Can you work these out from the model? Positions are in its coordinate system, mm. Face numbers are marked on the shaded views. Give positions to 0.01 mm unless a question says otherwise; leave off trailing zeros. Write each loop counter-clockwise with the first axis right and the second up, starting at its lowest first coordinate (ties: lowest second). Pieces come first, ordered by that corner, then holes.
from build123d import *

# Parameters (mm, degrees)
SKETCH1_R               = 17.5
BOSS_EXTRUDE1_DEPTH     = 15
SKETCH2_R               = 1.5
CUT_EXTRUDE1_DEPTH      = 3
CUT_EXTRUDE2_START      = -3
SKETCH3_R               = 1.5
CUT_EXTRUDE2_DEPTH      = 3
CUT_EXTRUDE3_DEPTH      = 0.2
CUT_EXTRUDE3_DEPTH_BACK = 0.2
SKETCH4_R               = 17.5
SKETCH4_R_2             = 16.5
CHAMFER1_SIZE           = 1
SKETCH5_R               = 2.5
CUT_EXTRUDE4_DEPTH      = 29.939592257


with BuildPart() as part:
    # Sketch1 → Boss-Extrude1 (new body)
    with BuildSketch(Plane(origin=(0, 0, 0), x_dir=(1, 0, 0), z_dir=(0, 1, 0))):
        with Locations(Location((0, 0, 0), (0, 0, 270))):
            Circle(SKETCH1_R)
    extrude(amount=BOSS_EXTRUDE1_DEPTH)

    # Sketch2 → Cut-Extrude1 (cut)
    with BuildSketch(Plane(origin=(0, 15, 0), x_dir=(1, 0, 0), z_dir=(0, 1, 0))):
        with Locations(Location((-8, 0, 0), (0, 0, 270))):
            Circle(SKETCH2_R)
        with Locations(Location((8, 0, 0), (0, 0, 270))):
            Circle(SKETCH2_R)
        with Locations(Location((0, 8, 0), (0, 0, 270))):
            Circle(SKETCH2_R)
        with Locations(Location((0, -8, 0), (0, 0, 270))):
            Circle(SKETCH2_R)
    extrude(amount=-CUT_EXTRUDE1_DEPTH, mode=Mode.SUBTRACT)

    # Sketch3 → Cut-Extrude2 (cut)
    with BuildSketch(Plane.XZ.offset(CUT_EXTRUDE2_START)):
        with Locations(Location((0, 9.5, 0), (0, 0, 270))):
            Circle(SKETCH3_R)
        with Locations(Location((0, -9.5, 0), (0, 0, 270))):
            Circle(SKETCH3_R)
        with Locations(Location((8, 0, 0), (0, 0, 90))):
            Circle(SKETCH3_R)
        with Locations(Location((-8, 0, 0), (0, 0, 90))):
            Circle(SKETCH3_R)
    extrude(amount=CUT_EXTRUDE2_DEPTH, mode=Mode.SUBTRACT)

    # Sketch4 → Cut-Extrude3 (cut, two sides: drawn at the far end of the back side and taken through both)
    with BuildSketch(Plane(origin=(0, 5, 0), x_dir=(-1, 0, 0), z_dir=(0, -1, 0)).offset(-CUT_EXTRUDE3_DEPTH_BACK)):
        with Locations(Location((0, 0, 0), (0, 0, 90))):
            Circle(SKETCH4_R)
        with Locations(Location((0, 0, 0), (0, 0, 90))):
            Circle(SKETCH4_R_2, mode=Mode.SUBTRACT)
    extrude(amount=CUT_EXTRUDE3_DEPTH + CUT_EXTRUDE3_DEPTH_BACK, mode=Mode.SUBTRACT)

    # Chamfer1
    chamfer1_edges = [part.edges().sort_by_distance(p)[0] for p in [
        (0, 0, -17.5),
        (0, 15, -17.5),
    ]]
    chamfer(chamfer1_edges, length=CHAMFER1_SIZE)

    # Sketch5 → Cut-Extrude4 (cut, through all)
    with BuildSketch(Plane(origin=(0, 15, 0), x_dir=(1, 0, 0), z_dir=(0, 1, 0))):
        with Locations(Location((0, 0, 0), (0, 0, 270))):
            Circle(SKETCH5_R)
    extrude(amount=-CUT_EXTRUDE4_DEPTH, mode=Mode.SUBTRACT)


solid = part.part
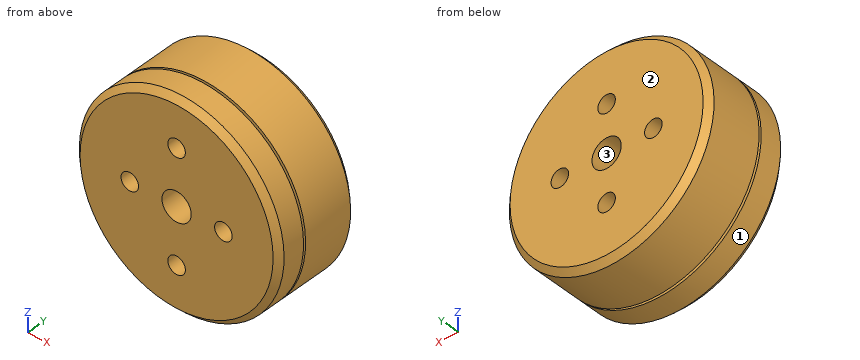
(1) If I drill on L1, parallel to X at y = 1.8, z = 0; L2, parallel to X at y = 12.7, z = -8; L3, parallel to X at y = 5.75, z = -1, over which ranges is the centre line in solid material (lowest first)?
Returned:
L1: x = -17.5 to -9.5, -6.5 to -2.5, 2.5 to 6.5, 9.5 to 17.5
L2: x = -15.56 to -1.5, 1.5 to 15.56
L3: x = -17.47 to -2.29, 2.29 to 17.47
(2) If we mould it in two halves opening along X, with no side actions, what happens to the marked faces 1, 2 and 3? For each: +X half, -X half, draft (parallel to the pull), parting line (faces both ways), or undercut.
Returned:
face 1: parting line
face 2: draft
face 3: undercut
(3) Imagine slicing it at A-A, the plane y = 11.5. Write out the boundary of the cut face in (x, z).
Returned:
outline: circle Ø35 at (0, 0); hole circle Ø5 at (0, 0)
(4) Will these pins go through, and if not, where does the flat tip stop? P1, Ø1.8, axis at x = -8, z = 0, coming from the +Y side; P2, Ø4.5, axis at x = 0, z = 0, coming from the -Y side; P3, Ø1.5, axis at y = 10, z = -4, coming from the -X side; P4, Ø2.5, axis at x = 8, z = 0, coming from the -Y side.
Returned:
P1: stops at y = 12
P2: passes through
P3: stops at x = -17.2
P4: stops at y = 3
